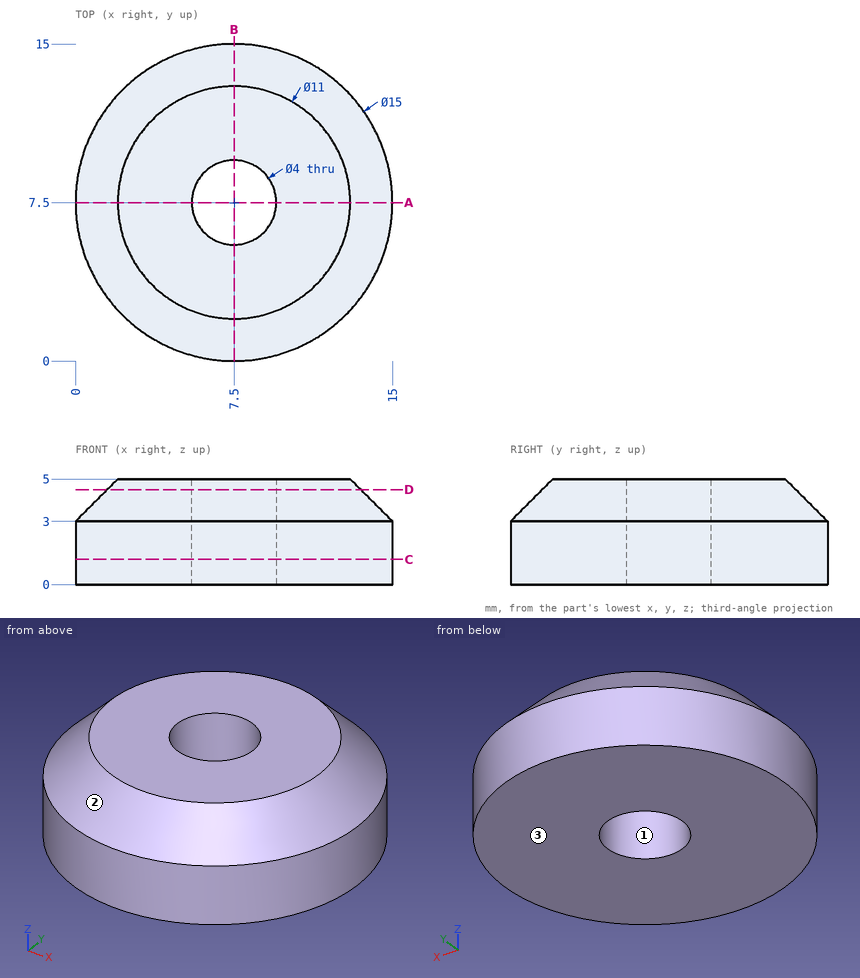
Here's the drawing with two shaded views (mm, measured from the low corner). I have some questions. Coordinates: 2 decimals unless noted, no trailing zeros. Write each loop counter-clockwise with the first axis right and the second up, starting at its lowest first coordinate (ties: lowest second). Pieces come first, ordered by that corner, then holes. Notation, with made-up numbers: (-30.75, -18) -> (-9.75, -18) arc R24 ccw to (-9.75, 13) -> close; hole circle Ø6 at (22, 82.25). An arc over 180 degrees is marked (long way). Write item = value, one per line. Start each with the question number.
(1) I want a section at C-C (z = 1.2). Please give me the cut outline in (x, y), plus the area to 3 significant figures.
(2) We'd pull the mould along X, two halves only. Please class the marked faces 1, 2 and 3: released by +X, released by -X, zero draft, split by the parting line, or undercut.
(3) I want a section at A-A (y = 7.5). Please give me the cut outline in (x, z), plus the area to 3 significant figures.
(4) Will this pin go through, and if not, where does the flat tip stop? pin 1 (1 mm diameter, centred on y = 6.5, z = 1, fed in from -X).
(5) I want a section at D-D (z = 4.5). Please give me the cut outline in (x, y), plus the area to 3 significant figures.
(6) I need wall thicknesses on line 1 (Y direction, x = 7.5, z = 2.8); line 2 (Y direction, x = 7.5, z = 3.65); line 3 (X direction, y = 7.25, z = 0.95). Which ranges of each line are inside material? Lowest first, please. Write a range as [from, to].
Result set:
q1.outline = circle Ø15 at (7.5, 7.5); hole circle Ø4 at (7.5, 7.5)
q1.area = 164 mm2
q2.face_1 = undercut
q2.face_2 = split by the parting line
q2.face_3 = zero draft
q3.outline = (0, 0) -> (5.5, 0) -> (5.5, 5) -> (2, 5) -> (0, 3) -> close; (9.5, 0) -> (15, 0) -> (15, 3) -> (13, 5) -> (9.5, 5) -> close
q3.area = 51.0 mm2
q4.pin_1 = 0.02
q5.outline = circle Ø12 at (7.5, 7.5); hole circle Ø4 at (7.5, 7.5)
q5.area = 101 mm2
q6.line_1 = [0, 5.5], [9.5, 15]
q6.line_2 = [0.65, 5.5], [9.5, 14.35]
q6.line_3 = [0, 5.52], [9.48, 15]
